Autodesk Fusion 360 part; units mm, degrees
sketch "Sketch1" plane through (0, 0, 0) normal (0, 1, 0) x (1, 0, 0)
  line L0 (0, 0) -> (0, 25)
  line L1 (0, 25) -> (3, 25)
  line L2 (3, 25) -> (3, 175.5)
  line L3 (3, 175.5) -> (88.5, 175.5)
  line L4 (88.5, 175.5) -> (88.5, 25)
  line L5 (88.5, 25) -> (30.5, 25)
  line L6 (30.5, 25) -> (30.5, 0)
  line L7 (30.5, 0) -> (34.5, 0)
  line L8 (34.5, 0) -> (34.5, 22)
  line L9 (34.5, 22) -> (91.5, 22)
  line L10 (91.5, 22) -> (91.5, 178.5)
  line L11 (91.5, 178.5) -> (0, 178.5)
  line L12 (0, 178.5) -> (0, 28)
  line L13 (0, 28) -> (-4, 28)
  line L14 (-4, 28) -> (-4, 0)
  line L15 (-4, 0) -> (0, 0)
  dimension "d1" = 4
  dimension "d2" = 3
  dimension "d3" = 3
  dimension "d4" = 3
  dimension "d5" = 3
  dimension "d6" = 3
  dimension "d7" = 4
  dimension "d8" = 85.5
  dimension "d9" = 150.5
  dimension "d10" = 25
  dimension "d11" = 25
  dimension "d12" = 3
  dimension "d13" = 30.5
extrude "Extrude1" add sketch "Sketch1" along normal blind 4
sketch "Sketch2" plane through (-4, 0, 0) normal (-1, 0, 0) x (0, 0, 1)
  line L0 (-28, 0) -> (0, 0)
  line L1 (0, 0) -> (0, 4)
  line L2 (0, 4) -> (-28, 4)
  line L3 (-28, 4) -> (-28, 0)
  line L4 (-25, 0) -> (-25, 4)
  circle A0 centre (-10, 4) radius 1.6
  line L5 (0, 4) -> (-7.5, 8.3301)
  line L6 (-12.5, 8.3301) -> (-20, 4)
  arc A1 (-7.5, 8.3301) -> (-12.5, 8.3301) centre (-10, 4) ccw
  point P0 (-25, 2)
  dimension "d16" = 3.2
  dimension "d17" = 10
  dimension "d18" = 2
  dimension "d19" = 15
  dimension "d20" = 30
extrude "Extrude2" add sketch "Sketch2" against normal up to surface (4 mm away) contours L2 A0 L5 L6 A1
extrude "Extrude3" add sketch "Sketch2" against normal up to surface (4 mm away) from surface at -34.5 contours L2 A0 L5 L6 A1
extrude "Extrude4" cut sketch "Sketch2" against normal through all contours L2 A0 picked at (-9.8813, 3.48)
fillet "Fillet1" radius 3 12 edges at (-2, 4, -20) (32.5, 4, -20) (32.5, 4, 0) (32.5, 0, 0) (-2, 4, 0) (-2, 0, 0) (-4, 2, -28) (0, 2, -28) (0, 2, -178.5) (91.5, 2, -178.5) (91.5, 2, -22) (34.5, 2, -22)
equation "d2 = d4"
equation "d3 = d4"
equation "d5 = d4"
equation "d6 = d4"
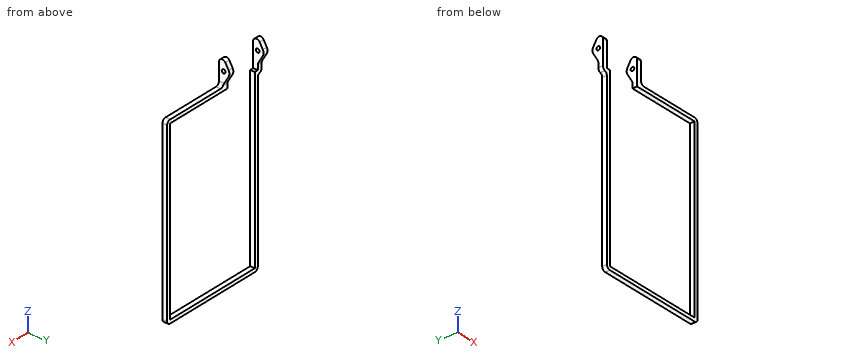
CAD build for the part. Positions are in the model's coordinates, mm. Coordinates: 2 decimals unless noted, no trailing zeros. Loops run counter-clockwise (first coordinate to the right, second up) from the corner with the lowest first, then second, coordinate; pieces in that order, holes last. Notation, with made-up numbers: (-21.75, 80.5) - (-17.75, 80.5) arc R23 cw to (-17.75, 115.5) - close; hole circle Ø2 at (13, -16.75). An arc over 180 degrees is marked (long way). Use CSV: the item, a comma, the result in double quotes. Start each with the question number.
Q1. Cut at C-C, the plane x = 13. List the corners of the cut face in (y, z), then the cut area to 3 significant figures.
Q2. Cut at A-A, the plane z = -163. List the corners of the cut face in (x, y).
Q3. Cut at B-B, the plane x = 59.5. List the corners of the cut face in (y, z).
Q4. Drop flat-ended pins along their axis: P1, Ø2, axis at y = 1, z = -114.5, coming from the -X side; P2, Ø4.5, axis at y = 3.5, z = -11, coming from the +X side; P3, Ø3, axis at x = 55, y = 1.5, coming from the +Z side. Give the stop position or say it passes through.
Q5. Probe probe 1 along Y at (x, z) = (-2.05, -10); probe 2 along X at (y, z) = (2.5, -59.5); probe 3 along Z at (x, y) = (62, 0.5). List the from-to ranges inside material, lowest first. Write a range as from..to.
Here are the results:
1,outline,"(0, -178.5) - (4, -178.5) - (4, -175.5) - (0, -175.5) - close"
1,area,"12.0 mm2"
2,outline,"(0, 0) - (3, 0) - (3, 4) - (0, 4) - close; (88.5, 0) - (91.5, 0) - (91.5, 4) - (88.5, 4) - close"
3,outline,"(0, -178.5) - (4, -178.5) - (4, -175.5) - (0, -175.5) - close; (0, -25) - (4, -25) - (4, -22) - (0, -22) - close"
4,P1,"x = 0"
4,P2,"x = 34.5"
4,P3,"z = -22"
5,probe 1,"0..2.4, 5.6..9"
5,probe 2,"0..3, 88.5..91.5"
5,probe 3,"-178.5..-175.5, -25..-22"
